Geometry check sheet. Reference: the model listing, model coordinates, mm. A direction names the side the tool comes from. Give positions to 0.01 mm unless a question says otherwise; leave off trailing zeros. Write each loop counter-clockwise with the first axis right and the second up, starting at its lowest first coordinate (ties: lowest second). Pieces come first, ordered by that corner, then holes. Notation, with made-up numbers: M 4,23.25 L 63,23.25 A12 ccw 63,39.25 Z; hole C 37,-20 d6. An arc over 180 degrees is marked long. One line per item, written item: value. Start each with the question number.
1. Cross-section at A-A on z = 3.75. Record the cut outline in (x, y), then the cut area to 3 significant figures.
2. Scan lines: line 1 (Y direction, x = 9, z = 5.1); line 2 (X direction, y = 6, z = 2.05); line 3 (Y direction, x = 9, z = 2.45). Record each from-to range of solid material in increasing order.
3. Gauge pin test, flat ends, axial feed: pin 1 (6 mm diameter, centred on x = 12, y = 5.5, fed in from +Z); pin 2 (1.9 mm diameter, centred on x = 8, y = 5, fed in from -Z); pin 3 (1.5 mm diameter, centred on y = 8.5, z = 4, fed in from +X); pin 4 (1 mm diameter, centred on x = 6.5, y = 5.5, fed in from -Z). Record the tip position at first contact, or that the pin passes through.
4. Release check for a two-part mould opening along X. For faces 3 (the face through (10.3, 4.6, 4.4)), 4 (the face through (8.89, 0.47, 0.48)), 5 (the face through (17, 10, 4)) record: pulls with the +X half, pulls with the -X half, needs draft (parallel to the pull), parting line crosses it, or undercut.
5. Cross-section at D-D on x = 12.25. Record the cut outline in (y, z).
6. Tool access check on faces 1 (the face through (10.4, 7.4, 4.4)), 2 (the face through (17.699, 0.285, 3.933)). Record the directions out of +Z, -Z, +X, -X, +Y, -Y that give a thin tool (end or side, any length) a straight path to the whole face; none if there is none.
7. Cross-section at C-C on x = 9.75. Record the cut outline in (y, z).
8. Cross-section at B-B on y = 5. Record the cut outline in (x, z).
from build123d import *

# Parameters (mm, degrees)
SKETCH_R     = 1.75
PAD_DEPTH    = 7
PAD001_DEPTH = 0.8
SKETCH002_R  = 3
POCKET_DEPTH = 4.4
SKETCH003_R  = 3
SKETCH003_W  = 3.5
SKETCH003_H  = 3.5
PAD002_DEPTH = 0.2
PAD003_DEPTH = 0.2
CHAMFER_SIZE = 0.95


with BuildPart() as part:
    # Sketch → Pad (new body)
    with BuildSketch(Plane.XY):
        with BuildLine():
            Line((18, 1), (18, 7))
            ThreePointArc((18, 7), (16.535534, 10.535534), (13, 12))
            Line((13, 12), (5, 12))
            ThreePointArc((5, 12), (1.464466, 10.535534), (0, 7))
            Line((0, 7), (0, 1))
            ThreePointArc((0, 1), (0.292893, 0.292893), (1, 0))
            Line((1, 0), (17, 0))
            ThreePointArc((17, 0), (17.707107, 0.292893), (18, 1))
        make_face()
        with Locations((9, 6)):
            Circle(SKETCH_R, mode=Mode.SUBTRACT)
    extrude(amount=PAD_DEPTH)

    # Sketch001 (on Face11 of Pad) → Pad001 (join)
    with BuildSketch(Plane.XY.offset(7)):
        with BuildLine():
            Line((6, 11.5), (6, 10.5))
            ThreePointArc((6, 10.5), (6.146447, 10.146447), (6.5, 10))
            Line((6.5, 10), (11.5, 10))
            ThreePointArc((11.5, 10), (11.853553, 10.146447), (12, 10.5))
            Line((12, 10.5), (12, 11.5))
            ThreePointArc((12, 11.5), (11.853553, 11.853553), (11.5, 12))
            Line((11.5, 12), (6.5, 12))
            ThreePointArc((6.5, 12), (6.146447, 11.853553), (6, 11.5))
        make_face()
        with BuildLine():
            Line((6, 1.5), (6, 0.5))
            ThreePointArc((6, 0.5), (6.146447, 0.146447), (6.5, 0))
            Line((6.5, 0), (11.5, 0))
            ThreePointArc((11.5, 0), (11.853553, 0.146447), (12, 0.5))
            Line((12, 0.5), (12, 1.5))
            ThreePointArc((12, 1.5), (11.853553, 1.853553), (11.5, 2))
            Line((11.5, 2), (6.5, 2))
            ThreePointArc((6.5, 2), (6.146447, 1.853553), (6, 1.5))
        make_face()
    extrude(amount=PAD001_DEPTH)

    # Sketch002 (on Face4 of Pad001) → Pocket (cut)
    with BuildSketch(Plane(origin=(0, 0, 0), x_dir=(1, 0, 0), z_dir=(0, 0, -1))):
        with Locations((9, -6)):
            Circle(SKETCH002_R)
    extrude(amount=-POCKET_DEPTH, mode=Mode.SUBTRACT)

    # Sketch003 (on Face29 of Pocket) → Pad002 (join)
    with BuildSketch(Plane(origin=(0, 0, 4.4), x_dir=(1, 0, 0), z_dir=(0, 0, -1))):
        with Locations((9, -6)):
            Circle(SKETCH003_R)
        with Locations((9, -6)):
            Rectangle(SKETCH003_W, SKETCH003_H, mode=Mode.SUBTRACT)
    extrude(amount=PAD002_DEPTH)

    # Sketch004 (on Face29 of Pad002) → Pad003 (join)
    with BuildSketch(Plane(origin=(0, 0, 4.2), x_dir=(1, 0, 0), z_dir=(0, 0, -1))):
        with BuildLine():
            ThreePointArc((11.436699, -4.25), (9, -3), (6.563301, -4.25))
            Line((6.563301, -4.25), (11.436699, -4.25))
        make_face()
        with BuildLine():
            ThreePointArc((6.563301, -7.75), (9, -9), (11.436699, -7.75))
            Line((6.563301, -7.75), (11.436699, -7.75))
        make_face()
    extrude(amount=PAD003_DEPTH)

    # Chamfer
    chamfer_edges = [part.edges().sort_by_distance(p)[0] for p in [
        (0.292893, 0.292893, 0),
    ]]
    chamfer(chamfer_edges, length=CHAMFER_SIZE)


solid = part.part
Report:
1. outline: M 0,1 A1 ccw 1,0 L 17,0 A1 ccw 18,1 L 18,7 A5 ccw 13,12 L 5,12 A5 ccw 0,7 Z; hole C 9,6 d6
1. area: 177 mm^2
2. line 1: y = 0 to 4.25, 7.75 to 12
2. line 2: x = 0 to 6, 12 to 18
2. line 3: y = 0 to 3, 9 to 12
3. pin 1: stops at z = 7
3. pin 2: stops at z = 4
3. pin 3: stops at x = 17.94
3. pin 4: stops at z = 0
4. face 3: undercut
4. face 4: needs draft
4. face 5: pulls with the +X half
5. outline: M 0,0.95 L 0.95,0 L 11.05,0 L 12,0.95 L 12,7 L 0,7 Z
6. face 1: -Z
6. face 2: +Z, -Z, +X, -Y
7. outline: M 0,0.95 L 0.95,0 L 3.1,0 L 3.1,4 L 4.25,4 L 4.25,4.4 L 4.42,4.4 L 4.42,7 L 2,7 L 2,7.8 L 0,7.8 Z; M 7.58,4.4 L 7.75,4.4 L 7.75,4 L 8.9,4 L 8.9,0 L 11.05,0 L 12,0.95 L 12,7.8 L 10,7.8 L 10,7 L 7.58,7 Z
8. outline: M 0,0.95 L 0.95,0 L 6.17,0 L 6.17,4.2 L 7.25,4.2 L 7.25,4.4 L 7.56,4.4 L 7.56,7 L 0,7 Z; M 10.44,4.4 L 10.75,4.4 L 10.75,4.2 L 11.83,4.2 L 11.83,0 L 17.05,0 L 18,0.95 L 18,7 L 10.44,7 Z
